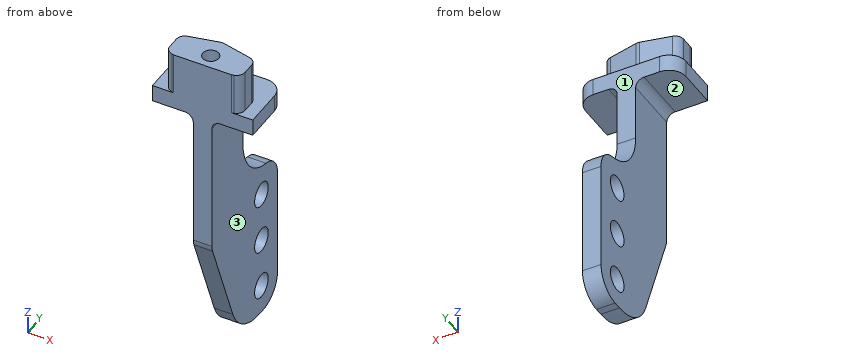
```python
from build123d import *

# Parameters (mm, degrees)
SKETCH3_W                      = 5.93
SKETCH3_H                      = 4.886
MOUNT_BASE_PLATE_DEPTH         = 1
HORN_LEVER_PROFILE_W           = 1.1
HORN_LEVER_PROFILE_H           = 7
LEVER_PROFILE_DEPTH            = 16.204
LOWER_CH_FRONT_DIVOT_W         = 6.814
LOWER_CH_FRONT_DIVOT_H         = 3.69
FRONT_BASE_PROFILE_CUT_DEPTH   = 19.667421273
REAR_PROFILE_CUT_DEPTH         = 19.667421273
F_3_HOLES_R                    = 0.7239
F_3_HOLES_CIUT_DEPTH           = 19.667421273
THRU_BASE_MOUNT_TAB_DEPTH      = 2.5
SKETCH9_R                      = 0.47117
THRU_BASE_MOUNT_TAB_HOLE_DEPTH = 4
BASE_PLATE_CORNER_FILLET_R     = 1
FRONT_LEVER_UNDER_FILLET_R     = 3
FRONT_LEVER_TOP_FILLETS_R      = 1.5
REAR_TOP_FILLET_R              = 3
SIDE_BASE_LEVER_ARM_FILLETS_R  = 0.5
THRU_BASE_MOUNT_TAB_FILLETS_R  = 0.5
BOT_MIIDLEVER_ANGLE_FILLET_R   = 1


with BuildPart() as part:
    # Sketch3 → Mount Base Plate (new body)
    with BuildSketch(Plane.XY):
        with Locations((0, 2.443)):
            Rectangle(SKETCH3_W, SKETCH3_H)
    extrude(amount=MOUNT_BASE_PLATE_DEPTH)

    # Horn Lever Profile → Lever Profile (add)
    with BuildSketch(Plane.XY):
        with Locations((0, 5.076)):
            Rectangle(HORN_LEVER_PROFILE_W, HORN_LEVER_PROFILE_H)
    extrude(amount=-LEVER_PROFILE_DEPTH)

    # Lower CH Front Divot → Front Base Profile Cut (cut, through all)
    with BuildSketch(Plane(origin=(0.55, 0, 0), x_dir=(0, 0, -1), z_dir=(1, 0, 0))):
        with Locations((3.407, 6.731)):
            Rectangle(LOWER_CH_FRONT_DIVOT_W, LOWER_CH_FRONT_DIVOT_H)
    extrude(amount=-FRONT_BASE_PROFILE_CUT_DEPTH, mode=Mode.SUBTRACT)

    # Sketch6 → Rear Profile Cut (cut, through all)
    with BuildSketch(Plane(origin=(0.55, 0, 0), x_dir=(0, 0, -1), z_dir=(1, 0, 0))):
        Polygon((8.434, 1.576), (16.204, 4.547737021), (16.204, 1.576), align=None)
    extrude(amount=-REAR_PROFILE_CUT_DEPTH, mode=Mode.SUBTRACT)

    # 3 Holes → 3 Holes Ciut (cut, through all)
    with BuildSketch(Plane(origin=(0.55, 0, 0), x_dir=(0, 0, -1), z_dir=(1, 0, 0))):
        with Locations(Location((14.4801, 6.8521, 0), (0, 0, 90))):
            Circle(F_3_HOLES_R)
        with Locations(Location((11.4801, 6.8521, 0), (0, 0, 90))):
            Circle(F_3_HOLES_R)
        with Locations(Location((8.4801, 6.8521, 0), (0, 0, 90))):
            Circle(F_3_HOLES_R)
    extrude(amount=-F_3_HOLES_CIUT_DEPTH, mode=Mode.SUBTRACT)

    # Thru Surface Base Ext → Thru Base Mount Tab (add)
    with BuildSketch(Plane.XY.offset(1)):
        Polygon((0, 3.693), (2.226, 3.193), (2.226, 1.693), (0, 1.193), (-2.226, 1.693), (-2.226, 3.193), align=None)
    extrude(amount=THRU_BASE_MOUNT_TAB_DEPTH)

    # Sketch9 → Thru Base Mount Tab Hole (cut)
    with BuildSketch(Plane.XY.offset(3.5)):
        with Locations((0, 2.443)):
            Circle(SKETCH9_R)
    extrude(amount=-THRU_BASE_MOUNT_TAB_HOLE_DEPTH, mode=Mode.SUBTRACT)

    # Base Plate Corner Fillet
    base_plate_corner_fillet_edges = [part.edges().sort_by_distance(p)[0] for p in [
        (-2.965, 4.886, 0.5),
        (2.965, 4.886, 0.5),
        (2.965, 0, 0.5),
        (-2.965, 0, 0.5),
    ]]
    fillet(base_plate_corner_fillet_edges, radius=BASE_PLATE_CORNER_FILLET_R)

    # Front Lever Under Fillet
    front_lever_under_fillet_edges = [part.edges().sort_by_distance(p)[0] for p in [
        (0, 4.886, -6.814),
    ]]
    fillet(front_lever_under_fillet_edges, radius=FRONT_LEVER_UNDER_FILLET_R)

    # Front Lever Top Fillets
    # the kernel refuses this fillet: 1.5 mm, written as the material it takes off along each edge
    with BuildSketch(Plane(origin=(4.3, 8.576, -16.204), x_dir=(0, 0, 1), z_dir=(-1, 0, 0))) as front_lever_top_fillets_piece_1:
        with BuildLine():
            CenterArc((FRONT_LEVER_TOP_FILLETS_R, -FRONT_LEVER_TOP_FILLETS_R), FRONT_LEVER_TOP_FILLETS_R, 90, 90)
            Line((0, -FRONT_LEVER_TOP_FILLETS_R), (0, 0))
            Line((0, 0), (FRONT_LEVER_TOP_FILLETS_R, 0))
        make_face()
    extrude(amount=8.6, mode=Mode.SUBTRACT)
    with BuildSketch(Plane(origin=(4.116249365, 8.576, -6.814), x_dir=(0, -0.9992074286085749, 0.03980596203384177), z_dir=(-1, 0, 0))) as front_lever_top_fillets_piece_2:
        with BuildLine():
            CenterArc((1.442027948, -1.485078086), FRONT_LEVER_TOP_FILLETS_R, 98.088443448, 79.630240195)
            Line((-0.056783195, -1.425369143), (-0.206664309, -1.419398249))
            Line((-0.206664309, -1.419398249), (-0.149881114, 0.005970894))
            Line((-0.149881114, 0.005970894), (0.005970894, 0.149881114))
            ThreePointArc((0.005970894, 0.149881114), (0.69542402, 0.122415), (1.209870405, 0.148507809))
            Line((1.209870405, 0.148507809), (1.230975636, 0))
        make_face()
    extrude(amount=8.232498729, mode=Mode.SUBTRACT)

    # Rear Top Fillet
    rear_top_fillet_edges = [part.edges().sort_by_distance(p)[0] for p in [
        (0, 4.547737021, -16.204),
    ]]
    fillet(rear_top_fillet_edges, radius=REAR_TOP_FILLET_R)

    # Side Base Lever Arm Fillets
    side_base_lever_arm_fillets_edges = [part.edges().sort_by_distance(p)[0] for p in [
        (-0.55, 3.231, 0),
        (0.55, 3.231, 0),
    ]]
    fillet(side_base_lever_arm_fillets_edges, radius=SIDE_BASE_LEVER_ARM_FILLETS_R)

    # Thru base Mount Tab Fillets
    thru_base_mount_tab_fillets_edges = [part.edges().sort_by_distance(p)[0] for p in [
        (0, 3.693, 2.25),
        (-2.226, 3.193, 2.25),
        (-2.226, 1.693, 2.25),
        (0, 1.193, 2.25),
        (2.226, 1.693, 2.25),
        (2.226, 3.193, 2.25),
    ]]
    fillet(thru_base_mount_tab_fillets_edges, radius=THRU_BASE_MOUNT_TAB_FILLETS_R)

    # Bot MiidLever Angle Fillet
    bot_miidlever_angle_fillet_edges = [part.edges().sort_by_distance(p)[0] for p in [
        (0, 1.576, -8.434),
    ]]
    fillet(bot_miidlever_angle_fillet_edges, radius=BOT_MIIDLEVER_ANGLE_FILLET_R)

    # SurfaceCut1
    split(bisect_by=Plane.XZ.offset(-1.576), keep=Keep.BOTTOM)


solid = part.part
```
Can you work these out from the model? Positions are in its coordinate system, mm. Face numbers are marked on the shaded views. A direction names the side the tool comes from. Round coordinates to 2 decimals unless told otherwise and drop trailing zeros. Order: outer loops, then holes, each group sorted by start corner. A loop starts at its lowest first (then second) coordinate and runs counter-clockwise, first axis right, second up.
(1) If I drill on L1, parallel to Y at x = 0.1, z = -0.75; L2, parallel to X at y = 5.5, z = -8.5; L3, parallel to Y at x = 0, z = 1.95, over which ranges is the centre line in solid material (lowest first)?
Results are:
L1: y = 1.58 to 4.89
L2: x = -0.55 to 0.55
L3: y = 1.58 to 1.97, 2.91 to 3.68
(2) If we section it at B-B (y = 4.25): Please give me the cut outline in (x, z).
Results are:
outline: (-2.9, 0) - (-1.05, 0) arc R0.5 cw to (-0.55, -0.5) - (-0.55, -15.05) - (0.55, -15.05) - (0.55, -0.5) arc R0.5 cw to (1.05, 0) - (2.9, 0) - (2.9, 1) - (-2.9, 1) - close
(3) I'm going to push flat-ended pins straight in: pin 1 (1.5 mm diameter, centred on x = 1, y = 7, fed in from +Z); pin 2 (3.5 mm diameter, centred on y = 6.5, z = -7, fed in from +X); pin 3 (2 mm diameter, centred on x = -0.5, z = -1, fed in from +Y); pin 4 (0.9 mm diameter, centred on y = 6.85, z = -14.48, fed in from +X). Where does each tip first touch, or does it pass through?
Results are:
pin 1: stops at z = -6.42
pin 2: stops at x = 0.55
pin 3: stops at y = 4.89
pin 4: passes through
(4) If we section it at A-A (z = 1.25): Please give me the cut outline in (x, y).
Results are:
outline: (-2.23, 2.09) arc R0.5 ccw to (-1.84, 1.61) - (-1.71, 1.58) - (1.71, 1.58) - (1.84, 1.61) arc R0.5 ccw to (2.23, 2.09) - (2.23, 2.79) arc R0.5 ccw to (1.84, 3.28) - (0.11, 3.67) arc R0.5 ccw to (-0.11, 3.67) - (-1.84, 3.28) arc R0.5 ccw to (-2.23, 2.79) - close; hole circle Ø0.94 at (0, 2.44)
(5) If we section it at C-C (x = -2.4): Please give me the cut outline in (y, z).
Results are:
outline: (1.58, 0) - (4.79, 0) - (4.79, 1) - (1.58, 1) - close
(6) On a 3-axis mill with a long thin cutter (end or side, diameter ignored), from which of +Z, -Z, +X, -X, +Y, -Y can I reach the whole of each face in a straight line? I mean the marked faces 1, 2 and 3. Say none if no direction works.
Results are:
face 1: +Z, +X, -X, +Y
face 2: -Z, -X, +Y, -Y
face 3: -Z, +X, +Y, -Y
(7) If we section it at D-D (z = -5): Please give me the cut outline in (x, y).
Results are:
outline: (-0.55, 1.58) - (0.55, 1.58) - (0.55, 5.13) - (-0.55, 5.13) - close
